Can you work these out from the model? Positions are in its coordinate system, mm. Give positions to 0.01 mm unless a question says otherwise; leave off trailing zeros. Order: outer loops, then holes, each group sorted by start corner. A loop starts at its lowest first (then second) coordinate and runs counter-clockwise, first axis right, second up. Notation, with made-up numbers: (25, 31) - (53, 31) arc R15 ccw to (53, 54) - close; hole circle Ø6 at (-10.5, 55). An arc over 180 degrees is marked (long way). Answer as CSV lines item,"result".
```python
from build123d import *

# Parameters (mm, degrees)
SKETCH1_R           = 1.375
BOSS_EXTRUDE1_DEPTH = 1.6
CUT_EXTRUDE1_DEPTH  = 0.1


with BuildPart() as part:
    # Sketch1 → Boss-Extrude1 (new body)
    with BuildSketch(Plane.XY):
        with BuildLine():
            Line((-39.5, -28), (39.5, -28))
            ThreePointArc((39.5, -28), (41.621320344, -27.121320344), (42.5, -25))
            Line((42.5, -25), (42.5, 25))
            ThreePointArc((42.5, 25), (41.621320344, 27.121320344), (39.5, 28))
            Line((39.5, 28), (-39.5, 28))
            ThreePointArc((-39.5, 28), (-41.621320344, 27.121320344), (-42.5, 25))
            Line((-42.5, 25), (-42.5, -25))
            ThreePointArc((-42.5, -25), (-41.621320344, -27.121320344), (-39.5, -28))
        make_face()
        with Locations((-39, 24.5)):
            Circle(SKETCH1_R, mode=Mode.SUBTRACT)
        with Locations((-39, -24.5)):
            Circle(SKETCH1_R, mode=Mode.SUBTRACT)
        with Locations((19, 24.5)):
            Circle(SKETCH1_R, mode=Mode.SUBTRACT)
        with Locations((19, -24.5)):
            Circle(SKETCH1_R, mode=Mode.SUBTRACT)
    extrude(amount=BOSS_EXTRUDE1_DEPTH)

    # Sketch2 → Cut-Extrude1 (cut)
    with BuildSketch(Plane.XY.offset(1.6)):
        Polygon((-35.65, -28.636850855), (-28.15, -28.636850855), (-28.15, -23.2), (-31.573707352, -23.2), (-31.573707352, -23.3), (-28.25, -23.3), (-28.25, -28.536850855), (-35.55, -28.536850855), (-35.55, -23.3), (-32.465045999, -23.3), (-32.465045999, -23.2), (-35.65, -23.2), align=None)
        Polygon((-17.75, -17.5), (-11.015830732, -17.5), (-11.015830732, -17.6), (-17.65, -17.6), (-17.65, -33.061376344), (-3.35, -33.061376344), (-3.35, -17.6), (-9.684859924, -17.6), (-9.684859924, -17.5), (-3.25, -17.5), (-3.25, -33.161376344), (-17.75, -33.161376344), align=None)
        Polygon((0.5, -5.3), (4.5, -5.3), (4.5, -27.7), (0.5, -27.7), (0.5, -17.125), (0.6, -17.125), (0.6, -27.6), (4.4, -27.6), (4.4, -5.4), (0.6, -5.4), (0.6, -15.17398131), (0.5, -15.17398131), align=None)
        Polygon((7.5, -15.5), (9.799158316, -15.5), (9.799158316, -15.6), (7.6, -15.6), (7.6, -31.061376344), (14.4, -31.061376344), (14.4, -15.6), (12.062610562, -15.6), (12.062610562, -15.5), (14.5, -15.5), (14.5, -31.161376344), (7.5, -31.161376344), align=None)
        Polygon((-35.45, 27), (15.45, 27), (15.45, 22), (-8.906687942, 22), (-8.906687942, 22.1), (15.35, 22.1), (15.35, 26.9), (-35.35, 26.9), (-35.35, 22.1), (-11.458179647, 22.1), (-11.458179647, 22), (-35.45, 22), align=None)
        Polygon((-41.371710411, -10.514157593), (-37.371710411, -10.514157593), (-37.371710411, 0.094714316), (-37.471710411, 0.094714316), (-37.471710411, -10.414157593), (-41.271710411, -10.414157593), (-41.271710411, 10.414157593), (-37.471710411, 10.414157593), (-37.471710411, 1), (-37.371710411, 1), (-37.371710411, 10.514157593), (-41.371710411, 10.514157593), align=None)
        Polygon((23.2, -25.5), (44.7, -25.5), (44.7, -10), (23.2, -10), (23.2, -16.5), (23.3, -16.5), (23.3, -10.1), (44.6, -10.1), (44.6, -25.4), (23.3, -25.4), (23.3, -17.75), (23.2, -17.75), align=None)
        Polygon((26.8, -5.5), (54.071370237, -5.5), (54.071370237, 7.5), (26.8, 7.5), (26.8, 2.552788505), (26.9, 2.552788505), (26.9, 7.4), (53.971370237, 7.4), (53.971370237, -5.4), (26.9, -5.4), (26.9, 0.407211154), (26.8, 0.407211154), align=None)
        Polygon((26.8, 12.5), (57.71374017, 12.5), (57.71374017, 25.5), (26.8, 25.5), (26.8, 20.277341759), (26.9, 20.277341759), (26.9, 25.4), (57.61374017, 25.4), (57.61374017, 12.6), (26.9, 12.6), (26.9, 18.611308355), (26.8, 18.611308355), align=None)
    extrude(amount=-CUT_EXTRUDE1_DEPTH, mode=Mode.SUBTRACT)


solid = part.part
```
1) I want a section at A-A on x = 19. Write out the boundary of the cut face in (y, z) (3 decimals), plus the area to 3 significant figures.
Answer block:
outline,"(-28, 0) - (-25.875, 0) - (-25.875, 1.6) - (-28, 1.6) - close; (-23.125, 0) - (23.125, 0) - (23.125, 1.6) - (-23.125, 1.6) - close; (25.875, 0) - (28, 0) - (28, 1.6) - (25.875, 1.6) - close"
area,"80.8 mm2"
2) If we mould it in two halves opening along X, with no side actions, what happens to faces 1 (the cylindrical face through (41.64, 27.1, 0.79)), 2 (the flat face through (-1, 0, 0)), 3 (the cylindrical face through (-40.013, -23.571, 0.789))? For each: +X half, -X half, draft (parallel to the pull), parting line (faces both ways), or undercut.
Answer block:
face 1,"+X half"
face 2,"draft"
face 3,"undercut"
3) I need wall thicknesses on line 1 along Y through (x, z) = (-39, 0.7) (3 decimals); line 2 along Y through (x, z) = (20, 1.4). Which ranges of each line are inside material? Lowest first, please. Write a range as [from, to].
Answer block:
line 1,"[-28, -25.875], [-23.125, 23.125], [25.875, 28]"
line 2,"[-28, -25.44], [-23.56, 23.56], [25.44, 28]"
